Read the model definition and answer for the solid it produces. Units are mm, in the model's axes. Coordinates: 2 decimals unless noted, no trailing zeros. Write each loop counter-clockwise with the first axis right and the second up, starting at its lowest first coordinate (ties: lowest second). Pieces come first, ordered by that corner, then holes.
(1) Find the intervals of material crossed by probe 1 along Y at (x, z) = (-48, -1); probe 2 along X at (y, z) = (1, -27.5); probe 3 along Y at (x, z) = (26.5, 3), in increasing order.
(2) Section B-B on x = -28.5 is taken. Write down the section's boundary in (y, z).
(3) Given pin 1 (11 mm diameter, centred on x = -32, z = -1, fed in from -Y); pin 2 (4.5 mm diameter, centred on y = 2, z = -38.5, fed in from +X); pin 3 (3 mm diameter, centred on x = -39.5, y = 1, fed in from -Z); pin 4 (2 mm diameter, centred on x = -8.5, z = -9, fed in from -Y), each flat-ended and moving along its own axis, determine where each tip first touches the part or whether it passes through.
(4) Section C-C on z = 30.5 is taken. Write down the section's boundary in (x, y), then the cut area to 3 significant figures.
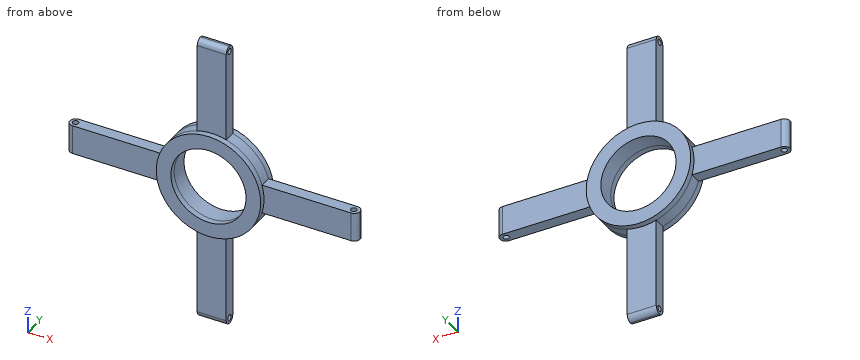
Autodesk Inventor part; units mm, degrees
ref_plane "YZ Plane" through (0, 0, 0) normal (1, 0, 0) x (0, 1, 0)
ref_plane "XZ Plane" through (0, 0, 0) normal (0, 1, 0) x (-1, 0, 0)
ref_plane "XY Plane" through (0, 0, 0) normal (0, 0, 1) x (1, 0, 0)
sketch "Boceto1" plane through (0, 0, 0) normal (0, 1, 0) x (-1, 0, 0)
  circle A0 centre (0, 0) radius 50 construction
  line L0 (-28.7316, 0) -> (21.6034, 0) construction
  circle A1 centre (0, 0) radius 12.95
  line L1 (50, 0) -> (-50, 0) construction
  line L2 (-50, 0) -> (-50, 5)
  line L3 (50, 5) -> (50, 0)
  line L4 (-50, 0) -> (-50, -5)
  line L5 (50, -5) -> (50, 0)
  line L6 (-50, -5) -> (-17.2916, -5)
  line L7 (17.2916, -5) -> (50, -5)
  line L8 (-50, 5) -> (-17.2916, 5)
  line L9 (17.2916, 5) -> (50, 5)
  line L10 (0, 50) -> (0, -50) construction
  line L11 (0, -50) -> (-5, -50)
  line L12 (-5, 50) -> (0, 50)
  line L13 (0, -50) -> (5, -50)
  line L14 (5, 50) -> (0, 50)
  arc A2 (-17.2916, -5) -> (-5, -17.2916) centre (0, 0) ccw
  arc A3 (5, -17.2916) -> (17.2916, -5) centre (0, 0) ccw
  arc A4 (17.2916, 5) -> (5, 17.2916) centre (0, 0) ccw
  arc A5 (-5, 17.2916) -> (-17.2916, 5) centre (0, 0) ccw
  line L15 (-5, -50) -> (-5, -17.2916)
  line L16 (-5, 17.2916) -> (-5, 50)
  line L17 (5, 17.2916) -> (5, 50)
  line L18 (5, -50) -> (5, -17.2916)
  dimension "d2" = 100
  dimension "d3" = 25.9
  dimension "d5" = 5
  dimension "d6" = 5
extrude "Extrusión1" add sketch "Boceto1" along normal blind 4
sketch "Boceto2" plane through (0, 4, 0) normal (0, 1, 0) x (1, 0, 0)
  circle A0 centre (0, 0) radius 18
  circle A1 centre (0, 0) radius 12.95
  dimension "d9" = 36
  dimension "d10" = 25.9
extrude "Extrusión2" add sketch "Boceto2" along normal blind 2
sketch "Boceto3" plane through (0, 0, 0) normal (0, -1, 0) x (1, 0, 0)
  circle A0 centre (0, 0) radius 18
  circle A1 centre (0, 0) radius 12.95
  dimension "d13" = 36
  dimension "d14" = 25.9
extrude "Extrusión3" add sketch "Boceto3" along normal blind 2
sketch "Boceto4" plane through (0, 4, 0) normal (0, 1, 0) x (1, 0, 0)
  point P0 (0, 0)
sketch "Boceto5" plane through (-5, 0, 50) normal (0, 0, 1) x (1, 0, 0)
  point P0 (5, 0)
sketch "Boceto6" plane through (-5, 0, 17.2916) normal (-1, 0, 0) x (0, 0, 1)
  line L0 (-67.2916, 4) -> (-63.2916, 4) construction
  line L1 (-63.2916, 4) -> (-63.2916, 0) construction
  line L2 (-63.2916, 0) -> (-67.2916, 0) construction
  line L3 (-67.2916, 0) -> (-67.2916, 4) construction
  line L4 (32.7084, 4) -> (0, 4) construction
  line L5 (32.7084, 4) -> (28.7084, 4)
  line L6 (28.7084, 4) -> (28.7084, 0) construction
  line L7 (28.7084, 0) -> (32.7084, 0) construction
  line L8 (32.7084, 0) -> (32.7084, 4) construction
  circle A0 centre (30.7084, 2) radius 1
  circle A1 centre (-65.2916, 2) radius 1
  point P0 (-17.2916, 0)
  dimension "d17" = 4
  dimension "d18" = 4
  dimension "d19" = 4
  dimension "d20" = 4
  dimension "d21" = 2
  dimension "d22" = 2
extrude "Extrusión4" cut sketch "Boceto6" against normal through all
sketch "Boceto7" plane through (17.2916, 0, 5) normal (0, 0, 1) x (1, 0, 0)
  line L0 (-34.5832, 4) -> (-67.2916, 4) construction
  line L1 (-67.2916, 4) -> (-63.2916, 4)
  line L2 (-63.2916, 4) -> (-63.2916, 0) construction
  line L3 (-63.2916, 0) -> (-67.2916, 0) construction
  line L4 (-67.2916, 0) -> (-67.2916, 4) construction
  circle A0 centre (-65.2916, 2) radius 1
  line L5 (32.7084, 4) -> (0, 4) construction
  line L6 (32.7084, 4) -> (28.7084, 4)
  line L7 (28.7084, 4) -> (28.7084, 0) construction
  line L8 (28.7084, 0) -> (32.7084, 0) construction
  line L9 (32.7084, 0) -> (32.7084, 4) construction
  circle A1 centre (30.5299, 2) radius 1
  point P0 (-17.2916, 0)
  dimension "d25" = 4
  dimension "d26" = 4
  dimension "d27" = 2
  dimension "d28" = 4
  dimension "d29" = 4
  dimension "d30" = 2
extrude "Extrusión5" cut sketch "Boceto7" against normal through all
fillet "Empalme1" radius 2 8 edges at (-50, 4, 0) (-50, 0, 0) (0, 4, 50) (0, 0, 50) (50, 4, 0) (50, 0, 0) (0, 4, -50) (0, 0, -50)
sketch "Boceto8" plane through (-17.2916, 0, 5) normal (0, 0, 1) x (1, 0, 0)
  point P0 (17.2916, 0)
sketch "Boceto9" plane through (5, 0, 17.2916) normal (1, 0, 0) x (0, 0, -1)
  point P0 (17.2916, 0)
Response:
1. probe 1: y = 0 to 1, 3 to 4
1. probe 2: x = -5 to 5
1. probe 3: y = 0 to 4
2. outline: (0, -5) - (4, -5) - (4, 5) - (0, 5) - close
3. pin 1: stops at y = 0
3. pin 2: stops at x = 5
3. pin 3: stops at z = -5
3. pin 4: stops at y = -2
4. outline: (-5, 0) - (5, 0) - (5, 4) - (-5, 4) - close
4. area: 40.0 mm2
